Can you work these out from the model? Positions are in its coordinate system, mm. Face numbers are marked on the shaded views. Round coordinates to 2 decimals unless told otherwise and drop trailing zeros. Loops run counter-clockwise (first coordinate to the right, second up) from the corner with the lowest first, then second, coordinate; pieces in that order, holes last. Notation, with made-up numbers: (-30.75, 82) -> (10.25, 82) arc R18 ccw to (10.25, 116) -> close; hole circle Ø1 at (22.25, 62.25). An arc over 180 degrees is marked (long way). Answer as a JSON object with one key per item and string values.
Autodesk Inventor part; units mm, degrees
ref_plane "YZ Plane" through (0, 0, 0) normal (1, 0, 0) x (0, 1, 0)
ref_plane "XZ Plane" through (0, 0, 0) normal (0, 1, 0) x (-1, 0, 0)
ref_plane "XY Plane" through (0, 0, 0) normal (0, 0, 1) x (1, 0, 0)
sketch "Sketch1" plane through (0, 0, 0) normal (0, 1, 0) x (-1, 0, 0)
  line L0 (5, 25) -> (-5, 25)
  line L1 (-5, 25) -> (-5, -25)
  line L2 (-5, -25) -> (5, -25)
  line L3 (5, -25) -> (5, 25)
  line L4 (5, 25) -> (-5, -25) construction
  line L5 (-5, 25) -> (5, -25) construction
  point P0 (0, 0)
  dimension "d0" = 10
  dimension "d1" = 50
extrude "Extrusion1" add sketch "Sketch1" along normal blind 2
sketch "Sketch2" plane through (0, 2, 0) normal (0, 1, 0) x (1, 0, 0)
  circle A0 centre (0, 18.75) radius 1.2
  line L0 (5, 25) -> (-5, 25)
  circle A1 centre (0, 12.5) radius 1.225
  circle A2 centre (0, 6.25) radius 1.25
  circle A3 centre (0, 0) radius 1.275
  circle A4 centre (0, -6.25) radius 1.3
  circle A5 centre (0, -12.5) radius 1.325
  circle A6 centre (0, -18.75) radius 1.35
  line L1 (0, 35) -> (0, -35)
  line L2 (-5, -25) -> (5, -25)
  dimension "d4" = 2.4
  dimension "d5" = 6.25
  dimension "d6" = 2.45
  dimension "d7" = 2.5
  dimension "d8" = 2.55
  dimension "d9" = 2.6
  dimension "d10" = 2.65
  dimension "d11" = 2.7
  dimension "d12" = 6.25
  dimension "d13" = 6.25
  dimension "d14" = 6.25
  dimension "d15" = 6.25
  dimension "d17" = 6.25
  dimension "d18" = 6.25
  dimension "d19" = 6.25
sketch "Sketch3" plane through (0, 2, 0) normal (0, 1, 0) x (1, 0, 0)
  line L0 (-5, -25) -> (5, -25)
  line L1 (5, -25) -> (5, 25)
  line L2 (5, 25) -> (-5, 25)
  line L3 (-5, 25) -> (-5, -25)
  circle A0 centre (0, 18.75) radius 1.2
  circle A1 centre (0, 18.75) radius 2.75
  circle A2 centre (0, 12.5) radius 2.75
  circle A3 centre (0, 6.25) radius 2.75
  circle A4 centre (0, 0) radius 2.75
  circle A5 centre (0, -6.25) radius 2.75
  circle A6 centre (0, -12.5) radius 2.75
  circle A7 centre (0, -18.75) radius 2.75
  dimension "d20" = 5.5
  dimension "d23" = 6.25
extrude "Extrusion2" add sketch "Sketch3" along normal blind 8 contours A0 | A1 | A2 | A3 | A4 | A5 | A6 | A7
extrude "Extrusion3" cut sketch "Sketch2" along normal blind 8
equation "\"d5\" = d19"
equation "\"d12\" = d5"
equation "\"d13\" = d5"
equation "\"d14\" = d5"
equation "\"d15\" = d5"
equation "\"d17\" = d5"
equation "\"d18\" = d5"
properties part number "test_gwintow"
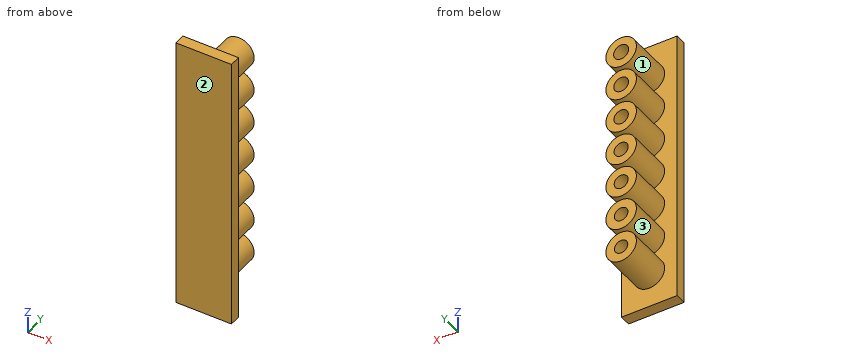
Q1. I want a section at C-C, the plane x = 3.75. Write out the boundary of the cut face in (y, z), then the cut area to 3 significant figures.
Determined:
{"outline": "(0, -25) -> (2, -25) -> (2, 25) -> (0, 25) -> close", "area": "100 mm²"}
Q2. We'd pull the mould along Z, two halves only. Please class the marked faces 1, 2 and 3: pulls with the +Z half, pulls with the -Z half, needs draft (parallel to the pull), parting line crosses it, or undercut.
Determined:
{"face 1": "undercut", "face 2": "needs draft", "face 3": "undercut"}
Q3. I want a section at A-A, the plane y = 2.5. Give the number of separate pieces and of enclosed holes in the cut face, then the cut area to 3 significant figures.
Determined:
{"separate pieces": "7", "enclosed holes": "7", "area": "131 mm²"}
Q4. I want a section at B-B, the plane z = 18.75. Write out the boundary of the cut face in (x, y), then the cut area to 3 significant figures.
Determined:
{"outline": "(-5, 0) -> (5, 0) -> (5, 2) -> (2.75, 2) -> (2.75, 10) -> (1.35, 10) -> (1.35, 2) -> (-1.35, 2) -> (-1.35, 10) -> (-2.75, 10) -> (-2.75, 2) -> (-5, 2) -> close", "area": "42.4 mm²"}
Q5. I'm going to push flat-ended pins straight in: pin 1 (1.5 mm diameter, centred on x = -1, y = 4.5, fed in from +Z); pin 2 (6 mm diameter, centred on x = -3.5, z = -6, fed in from +Y); pin 3 (1.5 mm diameter, centred on x = 1.5, y = 4.5, fed in from -Z); pin 4 (0.7 mm diameter, centred on x = 0.5, z = -13, fed in from +Y). Where does each tip first touch, or does it pass through?
Determined:
{"pin 1": "z = 21.49", "pin 2": "y = 10", "pin 3": "z = -21.4", "pin 4": "y = 2"}
Q6. If I drill on L1, parallel to X at y = 7.5, z = 12.5 (3 decimals); L2, parallel to X at y = 4.25, z = -18.75; L3, parallel to Y at x = -2, z = 15, over which ranges is the centre line in solid material (lowest first)? Write a range as [from, to].
Determined:
{"L1": "[-2.75, -1.325], [1.325, 2.75]", "L2": "[-2.75, -1.2], [1.2, 2.75]", "L3": "[0, 2]"}
Q7. I want a section at D-D, the plane z = -18.75. Write out the boundary of the cut face in (x, y).
Determined:
{"outline": "(-5, 0) -> (5, 0) -> (5, 2) -> (2.75, 2) -> (2.75, 10) -> (1.2, 10) -> (1.2, 2) -> (-1.2, 2) -> (-1.2, 10) -> (-2.75, 10) -> (-2.75, 2) -> (-5, 2) -> close"}
